```python
from build123d import *

# Parameters (mm, degrees)
BOSS_EXTRUDE1_DEPTH = 35
FILLET1_R           = 10
SHELL1_T            = -4
BOSS_EXTRUDE2_DEPTH = 2


with BuildPart() as part:
    # Sketch2 → Boss-Extrude1 (new body)
    with BuildSketch(Plane(origin=(0, 0, 0), x_dir=(1, 0, 0), z_dir=(0, 1, 0))):
        with BuildLine():
            Line((-29, 14), (29, 14))
            ThreePointArc((29, 14), (43, 0), (29, -14))
            Line((29, -14), (-29, -14))
            ThreePointArc((-29, -14), (-43, 0), (-29, 14))
        make_face()
    extrude(amount=BOSS_EXTRUDE1_DEPTH)

    # Fillet1
    fillet1_edges = [part.edges().sort_by_distance(p)[0] for p in [
        (43, 35, 0),
        (0, 35, -14),
        (-43, 35, 0),
        (0, 35, 14),
    ]]
    fillet(fillet1_edges, radius=FILLET1_R)

    # Shell1
    shell1_openings = [part.faces().sort_by_distance(p)[0] for p in [
        (0, 0, 0),
    ]]
    offset(amount=SHELL1_T, openings=shell1_openings, kind=Kind.INTERSECTION)

    # Sketch3 → Boss-Extrude2 (add)
    with BuildSketch(Plane.XZ):
        with BuildLine():
            Line((-29, -26), (29, -26))
            ThreePointArc((29, -26), (55, 0), (29, 26))
            Line((29, 26), (-29, 26))
            ThreePointArc((-29, 26), (-55, 0), (-29, -26))
        make_face()
        with BuildLine():
            Line((-29, -10), (29, -10))
            ThreePointArc((29, -10), (39, 0), (29, 10))
            Line((29, 10), (-29, 10))
            ThreePointArc((-29, 10), (-39, 0), (-29, -10))
        make_face(mode=Mode.SUBTRACT)
    extrude(amount=-BOSS_EXTRUDE2_DEPTH)


solid = part.part
```
Geometry check sheet. Reference: the model listing, model coordinates, mm. A direction names the side the tool comes from. Coordinates: 2 decimals unless noted, no trailing zeros. Order: outer loops, then holes, each group sorted by start corner. A loop starts at its lowest first (then second) coordinate and runs counter-clockwise, first axis right, second up.
Q1. Sectioned sample at B-B on x = 16. Record the cut outline in (y, z), and give its area (3 significant figures).
Reply:
outline: (0, -26) - (2, -26) - (2, -14) - (25, -14) arc R10 ccw to (35, -4) - (35, 4) arc R10 ccw to (25, 14) - (2, 14) - (2, 26) - (0, 26) - (0, 10) - (25, 10) arc R6 cw to (31, 4) - (31, -4) arc R6 cw to (25, -10) - (0, -10) - close
area: 381 mm2
Q2. Thickness scan on probe 1 along Z at (x, y) = (-11, 23.5); probe 2 along Z at (x, y) = (-5, 33); probe 3 along X at (y, z) = (8.5, -0.5). Record the ranges inside material, lowest first.
Reply:
probe 1: z = -14 to -10, 10 to 14
probe 2: z = -10 to 10
probe 3: x = -42.99 to -38.99, 38.99 to 42.99
Q3. Draft check along Z on faces 5 (the face through (-0.41, 31.99, 11.15)), 6 (the face through (39, 12, 0)), 7 (the face through (-1, 2, -17)). Enter one of: released by +Z, released by -Z, zero draft, split by the parting line, or undercut.
Reply:
face 5: released by +Z
face 6: undercut
face 7: zero draft
Q4. Sectioned sample at A-A on y = 11. Record the cut outline in (x, z).
Reply:
outline: (-29, -14) - (29, -14) arc R14 ccw to (29, 14) - (-29, 14) arc R14 ccw to start; hole (-29, -10) - (29, -10) arc R10 ccw to (29, 10) - (-29, 10) arc R10 ccw to start
Q5. Tool access check on faces 1 (the face through (0, 31, 0)), 2 (the face through (0, 13, 14)), 3 (the face through (-43, 13, 0)), 4 (the face through (0, 13, -14)). Record the directions out of +Z, -Z, +X, -X, +Y, -Y that give a thin tool (end or side, any length) a straight path to the whole face; none if there is none.
Reply:
face 1: -Y
face 2: +Z, +X, -X, +Y
face 3: -X, +Y
face 4: -Z, +X, -X, +Y
Q6. Depth check by flat-ended pin: pin 1 Ø18.5 at (x, y) = (-5.5, 11) entering from +Z; pin 2 Ø10 at (y, z) = (8.5, -12.5) entering from -X; pin 3 Ø4 at (x, z) = (-15, 0.5) entering from -Y; pin 4 Ø6 at (x, z) = (7, -10.5) entering from +Y. Enter the tip coordinate at first touch or a pass-through.
Reply:
pin 1: stops at z = 26
pin 2: stops at x = -40.82
pin 3: stops at y = 31
pin 4: stops at y = 34.37
Q7. Sectioned sample at C-C on z = -17. Record the cut outline in (x, y).
Reply:
outline: (-48.67, 0) - (48.67, 0) - (48.67, 2) - (-48.67, 2) - close
